Work out the finished part from the listing and answer in its coordinate system (mm). Give positions to 0.01 mm unless a question says otherwise; leave off trailing zeros. Write each loop counter-clockwise with the first axis right and the second up, starting at its lowest first coordinate (ties: lowest second). Pieces come first, ordered by that corner, then holes.
1) Find section B-B (z = 0). Determine the outline of the cut face in (x, y).
2) Find section C-C (z = 2.5). Determine the outline of the cut face in (x, y), plus the area to 3 significant figures.
3) Find section A-A (x = 0). Determine the outline of the cut face in (y, z).
4) Given pin 1 Ø2.5 at (x, z) = (0, -8) entering from +Y; pin 2 Ø3 at (y, z) = (3, -5) entering from +X; pin 3 Ø1.5 at (x, z) = (1, -6.5) entering from +Y; pin 4 Ø2 at (x, y) = (-5.5, 6) entering from -Z, each flat-ended and moving along its own axis, determine where each tip first touches the part or whether it passes through.
5) Straight lines are drawn through the part: probe 1 along X at (y, z) = (0.5, 0); probe 2 along Z at (x, y) = (0, 3.25); probe 3 along Y at (x, z) = (9.75, 3.5). For each, find the intervals that lie inside material, in ascending order.
6) Determine the mould class of faces 1 (the face through (1.5, 7.13, 4.77)), 2 (the face through (-5, 2.2, 2)), 3 (the face through (1.386, 6.625, -3.782)) for opening direction X: pulls with the +X half, pulls with the -X half, needs draft (parallel to the pull), parting line crosses it, or undercut.
7) Find section D-D (x = -8). Determine the outline of the cut face in (y, z), plus the area to 3 significant figures.
```python
from build123d import *

# Parameters (mm, degrees)
SKETCH_1_R               = 11
EXTRUDE_1_DEPTH          = 2.2
SKETCH_2_R               = 5
EXTRUDE_2_DEPTH          = 10
SKETCH_3_R               = 3
CUT_EXTRUDE_1_DEPTH      = 15
SKETCH_4_R               = 1.5
CUT_EXTRUDE_2_DEPTH      = 15
SKETCH_5_R               = 1.5
CUT_EXTRUDE_3_DEPTH      = 15
PATTERN_CIRCULAR_1_COUNT = 4


with BuildPart() as part:
    # Sketch 1 → Extrude 1 (new body)
    with BuildSketch(Plane(origin=(0, 0, 0), x_dir=(1, 0, 0), z_dir=(0, 1, 0))):
        with Locations(Location((0, 0, 0), (0, 0, 270))):
            Circle(SKETCH_1_R)
    extrude(amount=EXTRUDE_1_DEPTH)

    # Sketch 2 → Extrude 2 (add)
    with BuildSketch(Plane(origin=(0, 2.2, 0), x_dir=(1, 0, 0), z_dir=(0, 1, 0))):
        with Locations(Location((0, 0, 0), (0, 0, 270))):
            Circle(SKETCH_2_R)
    extrude(amount=EXTRUDE_2_DEPTH)

    # Sketch 3 → Cut-Extrude 1 (cut)
    with BuildSketch(Plane(origin=(0, 12.2, 0), x_dir=(1, 0, 0), z_dir=(0, 1, 0))):
        with Locations(Location((0, 0, 0), (0, 0, 270))):
            Circle(SKETCH_3_R)
    extrude(amount=-CUT_EXTRUDE_1_DEPTH, mode=Mode.SUBTRACT)

    # Sketch 4 → Cut-Extrude 2 (cut)
    with BuildSketch(Plane.XY):
        with Locations((0, 7.2)):
            Circle(SKETCH_4_R)
    extrude(amount=-CUT_EXTRUDE_2_DEPTH, mode=Mode.SUBTRACT)

    # Sketch 5 → Cut-Extrude 3 (cut)
    with BuildSketch(Plane(origin=(0, 2.2, 0), x_dir=(1, 0, 0), z_dir=(0, 1, 0))):
        with Locations(Location((-8, 0, 0), (0, 0, 270))):
            Circle(SKETCH_5_R)
    cut_extrude_3 = extrude(amount=-CUT_EXTRUDE_3_DEPTH, mode=Mode.SUBTRACT)

    # Pattern Circular 1: Cut-Extrude 3 ×4 about axis
    pattern_circular_1_axis = Axis((0, 0, 0), (0, 1, 0))
    for i in range(1, PATTERN_CIRCULAR_1_COUNT):
        add(cut_extrude_3.rotate(pattern_circular_1_axis, i * 360 / PATTERN_CIRCULAR_1_COUNT), mode=Mode.SUBTRACT)


solid = part.part
```
Results:
1. outline: (-11, 0) - (-9.5, 0) - (-9.5, 2.2) - (-11, 2.2) - close; (-6.5, 0) - (-3, 0) - (-3, 12.2) - (-5, 12.2) - (-5, 2.2) - (-6.5, 2.2) - close; (3, 0) - (6.5, 0) - (6.5, 2.2) - (5, 2.2) - (5, 12.2) - (3, 12.2) - close; (9.5, 0) - (11, 0) - (11, 2.2) - (9.5, 2.2) - close
2. outline: (-10.71, 0) - (-1.66, 0) - (-1.66, 12.2) - (-4.33, 12.2) - (-4.33, 2.2) - (-10.71, 2.2) - close; (1.66, 0) - (10.71, 0) - (10.71, 2.2) - (4.33, 2.2) - (4.33, 12.2) - (1.66, 12.2) - close
2. area: 93.3 mm2
3. outline: (0, -11) - (2.2, -11) - (2.2, -9.5) - (0, -9.5) - close; (0, -6.5) - (2.2, -6.5) - (2.2, -5) - (5.7, -5) - (5.7, -3) - (0, -3) - close; (0, 3) - (12.2, 3) - (12.2, 5) - (2.2, 5) - (2.2, 6.5) - (0, 6.5) - close; (0, 9.5) - (2.2, 9.5) - (2.2, 11) - (0, 11) - close; (8.7, -5) - (12.2, -5) - (12.2, -3) - (8.7, -3) - close
4. pin 1: passes through
4. pin 2: stops at x = 10.35
4. pin 3: stops at y = 2.2
4. pin 4: stops at z = -2.18
5. probe 1: x = -11 to -9.5, -6.5 to -3, 3 to 6.5, 9.5 to 11
5. probe 2: z = -5 to -3, 3 to 5
5. probe 3: y = 0 to 2.2
6. face 1: parting line crosses it
6. face 2: needs draft
6. face 3: undercut
7. outline: (0, -7.55) - (2.2, -7.55) - (2.2, -1.5) - (0, -1.5) - close; (0, 1.5) - (2.2, 1.5) - (2.2, 7.55) - (0, 7.55) - close
7. area: 26.6 mm2
